```python
from build123d import *

# Parameters (mm, degrees)
SKETCH1_R           = 10
BOSS_EXTRUDE1_DEPTH = 20
CUT_EXTRUDE1_START  = -17
CUT_EXTRUDE1_DEPTH  = 17
CIRPATTERN1_COUNT   = 8
BOSS_EXTRUDE2_START = 12
SKETCH3_R           = 10
BOSS_EXTRUDE2_DEPTH = 12
SKETCH4_W           = 22
SKETCH4_H           = 22
BOSS_EXTRUDE3_DEPTH = 3


with BuildPart() as part:
    # Sketch1 → Boss-Extrude1 (new body)
    with BuildSketch(Plane.XY):
        Circle(SKETCH1_R)
    extrude(amount=BOSS_EXTRUDE1_DEPTH)

    # Sketch2 → Cut-Extrude1 (cut)
    with BuildSketch(Plane.XY.offset(20).offset(CUT_EXTRUDE1_START)):
        with BuildLine():
            Line((-1.736481777, 9.84807753), (-1.389185421, 7.878462024))
            ThreePointArc((-1.389185421, 7.878462024), (0, 8), (1.389185421, 7.878462024))
            Line((1.389185421, 7.878462024), (1.736481777, 9.84807753))
            ThreePointArc((1.736481777, 9.84807753), (0, 10), (-1.736481777, 9.84807753))
        make_face()
    cut_extrude1 = extrude(amount=CUT_EXTRUDE1_DEPTH, mode=Mode.SUBTRACT)

    # CirPattern1: Cut-Extrude1 ×8 about axis
    cirpattern1_axis = Axis((0, 0, 0), (0, 0, 1))
    for i in range(1, CIRPATTERN1_COUNT):
        add(cut_extrude1.rotate(cirpattern1_axis, i * 360 / CIRPATTERN1_COUNT), mode=Mode.SUBTRACT)

    # Sketch3 → Boss-Extrude2 (add)
    with BuildSketch(Plane(origin=(0, 0, 0), x_dir=(-1, 0, 0), z_dir=(0, 0, -1)).offset(BOSS_EXTRUDE2_START)):
        Circle(SKETCH3_R)
    extrude(amount=-BOSS_EXTRUDE2_DEPTH)

    # Sketch4 → Boss-Extrude3 (add)
    with BuildSketch(Plane(origin=(0, 0, -12), x_dir=(-1, 0, 0), z_dir=(0, 0, -1))):
        Rectangle(SKETCH4_W, SKETCH4_H)
    extrude(amount=BOSS_EXTRUDE3_DEPTH)


solid = part.part
```
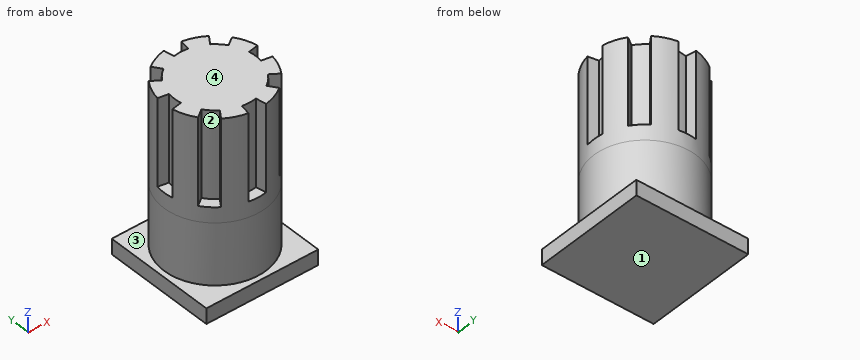
Geometry: final body of the model. Coordinates: model frame, mm. Face numbers are marked on the shaded views. A direction names the side the tool comes from. Round coordinates to 2 decimals unless told otherwise and drop trailing zeros. Loops run counter-clockwise (first coordinate to the right, second up) from the corner with the lowest first, then second, coordinate; pieces in that order, holes last. Notation, with made-up numbers: (-25.5, -19) -> (4.5, -19) arc R21 cw to (4.5, 14) -> close; hole circle Ø3 at (71, 38.25). An arc over 180 degrees is marked (long way). Use one line per item in the form item = value. Start each with the question number.
1) Access query for the marked faces 3 and 4. Directions: +Z, -Z, +X, -X, +Y, -Y. A direction counts if a zero-diameter tool reaches every point of the face in a straight line with its end or side. Return the directions, or none.
2) Section B-B on y = 0. Output: boundary loops of the cut face in (x, z).
3) Section D-D on y = -4. Output: boundary loops of the cut face in (x, z).
4) Line query: L1, parallel to Y at x = -5, z = 15 (3 decimals); L2, parallel to Z at x = 5, y = 10; L3, parallel to X at y = 6, z = -0.5. Output: solid intervals per line, ascending.
5) First-contact query: P1, Ø1.1, axis at x = -9, y = 0, coming from the +Z side; P2, Ø1, axis at x = -4.5, z = -3, coming from the -Y side; P3, Ø3, axis at y = 7, z = 12, coming from the -X side. Flat tips, straight axial feed; report the tip coordinate or a pass-through.
6) Draft query along Y for the marked faces 1 and 2. Return one class per face: released by +Y, released by -Y, zero draft, split by the parting line, or undercut.
Response:
q1.face_3 = +Z
q1.face_4 = +Z, +X, -X, +Y, -Y
q2.outline = (-11, -15) -> (11, -15) -> (11, -12) -> (10, -12) -> (10, 3) -> (8, 3) -> (8, 20) -> (-8, 20) -> (-8, 3) -> (-10, 3) -> (-10, -12) -> (-11, -12) -> close
q3.outline = (-11, -15) -> (11, -15) -> (11, -12) -> (9.17, -12) -> (9.17, 20) -> (-9.17, 20) -> (-9.17, -12) -> (-11, -12) -> close
q4.L1 = -8.66 to -7.141, -6.245 to 6.245, 7.141 to 8.66
q4.L2 = -15 to -12
q4.L3 = -8 to 8
q5.P1 = 3
q5.P2 = -9.17
q5.P3 = -8.35
q6.face_1 = zero draft
q6.face_2 = undercut
